The listing builds one solid part. Answer for the finished solid, in the listing's coordinates (mm). A direction names the side the tool comes from. Give positions to 0.01 mm unless a question says otherwise; leave off trailing zeros. Loops run counter-clockwise (first coordinate to the right, second up) from the corner with the lowest first, then second, coordinate; pieces in that order, holes last.
Item 1: Section A-A, the plane x = -10 is taken. Give the vertices of the cut face in (y, z), and give its area (3 significant figures).
Item 2: Each of these flat-tipped pins is pushed along its axis until it touches: pin 1 Ø4 at (y, z) = (10, 21) entering from +X; pin 2 Ø6.5 at (x, y) = (-9, 8) entering from +Z; pin 3 Ø8 at (x, z) = (-19, 5.5) entering from +Y. Where does it stop, or does it pass through?
Item 3: Section B-B, the plane x = -20.5 is taken. Give the vertices of the cut face in (y, z).
Item 4: The mould has two halves that part along X. Classify faces 1 (the face through (0, 13, 2)), 2 (the face through (-8, 8, 2)), 3 (the face through (-9.19, 9.05, 0.99)), 4 (the face through (-21, 3.5, 12)): pulls with the +X half, pulls with the -X half, needs draft (parallel to the pull), parting line crosses it, or undercut.
Item 5: Section D-D, the plane y = 4 is taken. Give the vertices of the cut face in (x, z), and give its area (3 significant figures).
Item 6: Section C-C, the plane y = 7.5 is taken. Give the vertices of the cut face in (x, z).
Item 7: Consider line 1 along Y through (x, z) = (-22.15, 32); line 2 along Y through (x, z) = (-10, 3.3); line 3 along X through (y, z) = (5.25, 13). Determine where each line is inside the solid, lowest interval first.
Item 8: A tool of negligible diameter and unlimited length cuts with its end or side. For faces 5 (the face through (13.25, 7, 2)), 6 (the face through (0, 2, 2)), 7 (the face through (-21, 11.5, 12)), from which of +Z, -Z, +X, -X, +Y, -Y can it reach the whole face along a straight path? Write none if from no direction.
Autodesk Inventor part; units mm, degrees
ref_plane "YZ Plane" through (0, 0, 0) normal (1, 0, 0) x (0, 1, 0)
ref_plane "XZ Plane" through (0, 0, 0) normal (0, 1, 0) x (-1, 0, 0)
ref_plane "XY Plane" through (0, 0, 0) normal (0, 0, 1) x (1, 0, 0)
sketch "Sketch1" plane through (0, 0, 0) normal (0, 0, 1) x (1, 0, 0)
  line L0 (0, 15) -> (20, 15)
  line L1 (20, 15) -> (20, 0)
  line L2 (20, 0) -> (0, 0)
  line L3 (0, 0) -> (0, 15)
  line L4 (3.25, 13) -> (6.75, 13)
  line L5 (6.75, 13) -> (6.75, 2)
  line L6 (6.75, 2) -> (3.25, 2)
  line L7 (3.25, 2) -> (3.25, 13)
  line L8 (13.25, 13) -> (16.75, 13)
  line L9 (16.75, 13) -> (16.75, 2)
  line L10 (16.75, 2) -> (13.25, 2)
  line L11 (13.25, 2) -> (13.25, 13)
  line L12 (0, 11.5) -> (-25, 11.5)
  line L13 (-25, 11.5) -> (-25, 3.5)
  line L14 (-25, 3.5) -> (0, 3.5)
  line L15 (0, 3.5) -> (0, 11.5)
  circle A0 centre (-10, 7.5) radius 1.75
  point P0 (0, -23)
  point P1 (0, 7.5)
  dimension "d0" = 20
  dimension "d1" = 2
  dimension "d2" = 2
  dimension "d3" = 3.5
  dimension "d4" = 3.25
  dimension "d5" = 6.5
  dimension "d6" = 3.5
  dimension "d8" = 15
  dimension "d9" = 25
  dimension "d10" = 8
  dimension "d22" = 3.5
  dimension "d23" = 10
extrude "Extrusion1" add sketch "Sketch1" along normal blind 5
sketch "Sketch2" plane through (0, 0, 5) normal (0, 0, 1) x (1, 0, 0)
  line L0 (-25, 3.5) -> (0, 3.5)
  line L1 (-25, 11.5) -> (-20, 11.5)
  line L2 (-20, 11.5) -> (-20, 3.5)
  line L3 (-20, 3.5) -> (-25, 3.5)
  line L4 (-25, 3.5) -> (-25, 11.5)
  dimension "d24" = 5
extrude "Extrusion2" add sketch "Sketch2" along normal blind 30
sketch "Sketch3" plane through (-25, 3.5, 0) normal (-1, 0, 0) x (0, 0, 1)
  line L0 (35, 8) -> (35, 0)
  circle A0 centre (32, 4) radius 1.75
  point P0 (0, -3.5)
  point P1 (35, 4)
  dimension "d17" = 3.5
  dimension "d18" = 3
extrude "Extrusion3" cut sketch "Sketch3" against normal blind 35
fillet "Fillet1" radius 3 2 edges at (-22.5, 11.5, 35) (-22.5, 3.5, 35)
sketch "Sketch4" plane through (0, 0, 5) normal (0, 0, 1) x (1, 0, 0)
  circle A0 centre (-10, 7.5) radius 1.75
  circle A1 centre (-10, 7.5) radius 3
  dimension "d26" = 6
extrude "Extrusion4" cut sketch "Sketch4" against normal blind 3
equation "\"d2\" = d1"
equation "\"d6\" = d3"
properties part number "switch bracket v5.1"
Worked answers:
1. outline: (3.5, 0) - (5.75, 0) - (5.75, 2) - (4.5, 2) - (4.5, 5) - (3.5, 5) - close; (9.25, 0) - (11.5, 0) - (11.5, 5) - (10.5, 5) - (10.5, 2) - (9.25, 2) - close
1. area: 15.0 mm2
2. pin 1: stops at x = -20
2. pin 2: stops at z = 5
2. pin 3: stops at y = 11.5
3. outline: (3.5, 0) - (11.5, 0) - (11.5, 32) arc R3 ccw to (8.5, 35) - (6.5, 35) arc R3 ccw to (3.5, 32) - close; hole circle Ø3.5 at (7.5, 32)
4. face 1: pulls with the -X half
4. face 2: undercut
4. face 3: undercut
4. face 4: needs draft
5. outline: (-25, 0) - (3.25, 0) - (3.25, 5) - (-20, 5) - (-20, 33.66) - (-25, 33.66) - close; (6.75, 0) - (13.25, 0) - (13.25, 5) - (6.75, 5) - close; (16.75, 0) - (20, 0) - (20, 5) - (16.75, 5) - close
5. area: 333 mm2
6. outline: (-25, 0) - (-11.75, 0) - (-11.75, 2) - (-13, 2) - (-13, 5) - (-20, 5) - (-20, 30.25) - (-25, 30.25) - close; (-25, 33.75) - (-20, 33.75) - (-20, 35) - (-25, 35) - close; (-8.25, 0) - (3.25, 0) - (3.25, 5) - (-7, 5) - (-7, 2) - (-8.25, 2) - close; (6.75, 0) - (13.25, 0) - (13.25, 5) - (6.75, 5) - close; (16.75, 0) - (20, 0) - (20, 5) - (16.75, 5) - close
7. line 1: y = 3.5 to 5.75, 9.25 to 11.5
7. line 2: y = 3.5 to 4.5, 10.5 to 11.5
7. line 3: x = -25 to -20
8. face 5: +Z, -Z
8. face 6: +Z, -Z, -X, -Y
8. face 7: +Z, -Z, -X, +Y
